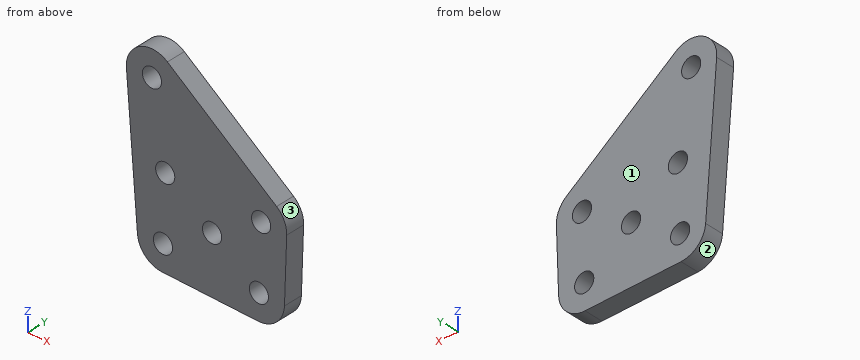
```python
from build123d import *

# Parameters (mm, degrees)
SKETCH1_R           = 1.5
BOSS_EXTRUDE1_DEPTH = 3


with BuildPart() as part:
    # Sketch1 → Boss-Extrude1 (new body)
    with BuildSketch(Plane(origin=(0, 0, 0), x_dir=(1, 0, 0), z_dir=(0, 1, 0))):
        with BuildLine():
            Line((-21.220362367, -4.8401676), (-38.281803408, -17.761164033))
            ThreePointArc((-38.281803408, -17.761164033), (-42.613403289, -18.083291405), (-44.684930136, -14.265530269))
            Line((-44.684930136, -14.265530269), (-42.961821092, 8.128352288))
            ThreePointArc((-42.961821092, 8.128352288), (-41.741950615, 10.708740743), (-39.11256419, 11.819063031))
            Line((-39.11256419, 11.819063031), (-24.121617673, 12.340141252))
            ThreePointArc((-24.121617673, 12.340141252), (-21.254198948, 11.26753095), (-19.985077742, 8.481509707))
            Line((-19.985077742, 8.481509707), (-19.637692261, -1.512454638))
            ThreePointArc((-19.637692261, -1.512454638), (-20.023012527, -3.36941295), (-21.220362367, -4.8401676))
        make_face()
        with Locations((-23.635277999, -1.65140883)):
            Circle(SKETCH1_R, mode=Mode.SUBTRACT)
        with Locations((-31.304443998, 3.085034231)):
            Circle(SKETCH1_R, mode=Mode.SUBTRACT)
        with Locations((-23.98266348, 8.342555514)):
            Circle(SKETCH1_R, mode=Mode.SUBTRACT)
        with Locations((-38.973609998, 7.821477293)):
            Circle(SKETCH1_R, mode=Mode.SUBTRACT)
        with Locations((-38.626224517, -2.172487052)):
            Circle(SKETCH1_R, mode=Mode.SUBTRACT)
        with Locations((-40.696719041, -14.572405264)):
            Circle(SKETCH1_R, mode=Mode.SUBTRACT)
    extrude(amount=BOSS_EXTRUDE1_DEPTH)


solid = part.part
```
Can you work these out from the model? Positions are in its coordinate system, mm. Face numbers are marked on the shaded views. Round coordinates to 2 decimals unless told otherwise and drop trailing zeros. Order: outer loops, then holes, each group sorted by start corner. A loop starts at its lowest first (then second) coordinate and runs counter-clockwise, first axis right, second up. Notation, with made-up numbers: (60.25, 10.25) -> (75.25, 10.25) arc R4 ccw to (75.25, 16.25) -> close; hole circle Ø3 at (-36, 53). An arc over 180 degrees is marked (long way). Return JSON: item names as keys, results as strings. Group by question number.
1. Will these pins go through, and if not, where does the flat tip stop? pin 1 (1 mm diameter, centred on y = 2.5, z = -4, fed in from +X); pin 2 (1.5 mm diameter, centred on y = 2, z = 8.5, fed in from +X).
2. We'd pull the mould along X, two halves only. Please class the marked faces 1, 2 and 3: released by +X, released by -X, zero draft, split by the parting line, or undercut.
3. If we section it at B-B, the plane y = 1.5: Write out the boundary of the cut face in (x, z).
4. If we section it at C-C, the plane x = -23.75: Write out the boundary of the cut face in (y, z), then the cut area to 3 significant figures.
5. If we section it at A-A, the plane z = -2.5: Write out the boundary of the cut face in (x, y), then the cut area to 3 significant figures.
6. If we section it at D-D, the plane z = 2.5: Write out the boundary of the cut face in (x, y), then the cut area to 3 significant figures.
7. I need wall thicknesses on line 1 (Z direction, x = -39.75, y = 2.35); line 2 (Z direction, x = -23, y = 1.45); line 3 (X direction, y = 2.6, z = -8). Which ranges of each line are inside material? Lowest first, please. Write a range as [from, to].
Output values:
{
 "1": {"pin 1": "x = -19.81", "pin 2": "x = -25.06"},
 "2": {"face 1": "zero draft", "face 2": "released by -X", "face 3": "released by +X"},
 "3": {"outline": "(-44.68, 14.27) -> (-42.96, -8.13) arc R4 ccw to (-39.11, -11.82) -> (-24.12, -12.34) arc R4 ccw to (-19.99, -8.48) -> (-19.64, 1.51) arc R4 ccw to (-21.22, 4.84) -> (-38.28, 17.76) arc R4 ccw to start; hole circle Ø3 at (-40.7, 14.57); hole circle Ø3 at (-38.97, -7.82); hole circle Ø3 at (-38.63, 2.17); hole circle Ø3 at (-31.3, -3.09); hole circle Ø3 at (-23.98, -8.34); hole circle Ø3 at (-23.64, 1.65)"},
 "4": {"outline": "(0, -12.34) -> (3, -12.34) -> (3, -9.82) -> (0, -9.82) -> close; (0, -6.86) -> (3, -6.86) -> (3, 0.16) -> (0, 0.16) -> close; (0, 3.15) -> (3, 3.15) -> (3, 6.76) -> (0, 6.76) -> close", "area": "39.4 mm²"},
 "5": {"outline": "(-43.39, 0) -> (-32.69, 0) -> (-32.69, 3) -> (-43.39, 3) -> close; (-29.92, 0) -> (-19.78, 0) -> (-19.78, 3) -> (-29.92, 3) -> close", "area": "62.6 mm²"},
 "6": {"outline": "(-43.78, 0) -> (-40.09, 0) -> (-40.09, 3) -> (-43.78, 3) -> close; (-37.16, 0) -> (-24.87, 0) -> (-24.87, 3) -> (-37.16, 3) -> close; (-22.4, 0) -> (-19.73, 0) -> (-19.73, 3) -> (-22.4, 3) -> close", "area": "56.0 mm²"},
 "7": {"line 1": "[-11.75, -9.1], [-6.54, 1.18], [3.17, 13.41], [15.74, 18.46]", "line 2": "[-12.22, -9.48], [-7.21, 0.29], [3.01, 6.19]", "line 3": "[-42.97, -40.46], [-37.48, -25.44], [-22.52, -19.97]"}
}
